Build history of the part. All positions in model axes, mm. A direction names the side the tool comes from. Round coordinates to 2 decimals unless told otherwise and drop trailing zeros. Order: outer loops, then holes, each group sorted by start corner. A loop starts at its lowest first (then second) coordinate and runs counter-clockwise, first axis right, second up. Notation, with made-up numbers: (68.5, 11.5) -> (88.5, 11.5) arc R20 ccw to (88.5, 41.5) -> close; hole circle Ø10 at (76, -27). An arc over 180 degrees is marked (long way). Use a Markdown table: item, result. Add a question column.
Item 1: Two-plate mould, pull along X, no slides. Class faces 5 (the face through (-2.3, 2, -15)), 6 (the face through (-20.94, 1.99, -0.69)), 7 (the face through (19.706, 1.993, -7.112)): released by +X, released by -X, zero draft, split by the parting line, or undercut.
Item 2: Probe L1, parallel to Z at x = -0.5, y = -0.3; L2, parallel to Z at x = -2.5, y = 1; L3, parallel to Z at x = 5, y = 1.9. List the from-to ranges inside material, lowest first.
Item 3: Slice it at C-C, the plane x = 0. State how many separate pieces and enclosed holes the cut face has, plus the area to 3 significant figures.
Item 4: Slice it at D-D, the plane y = -0.6. Give the cut face in (x, z), plus the area to 3 significant figures.
Item 5: 3-axis set-ups, long thin cutter, end or side, ignore diameter. For faces 1 (the face through (-8.53, -0.28, -8.44)), 2 (the face through (19.68, 1.99, 7.18)), 3 (the face through (15, 2, 4.796)), 4 (the face through (3.3, 2, 16)): which of +Z, -Z, +X, -X, +Y, -Y reach the whole face in a straight line?
Item 6: Pin check, flat tips, straight feed: pin 1 (2 mm diameter, centred on x = -3.5, y = 0, fed in from +Z); pin 2 (1.2 mm diameter, centred on x = -2, y = 0, fed in from +Z); pin 3 (19.5 mm diameter, centred on x = -3.5, z = 0.5, fed in from +Y); pin 4 (3 mm diameter, centred on x = 8, z = -14.5, fed in from -Y). Stop position of each tip, or through.
Item 7: Slice it at A-A, the plane x = -17. Give the cut face in (y, z).
from build123d import *

# Parameters (mm, degrees)
SKETCH2_W               = 4.6
SKETCH2_H               = 1.8
WATCH_POSITIONER_DEPTH  = 1
WATCH_HOLDER_V2_DEPTH   = 4
CHAMFER1_SIZE           = 0.6
CUT_EXTRUDE1_DEPTH      = 30.733062405
CUT_EXTRUDE1_DEPTH_BACK = 30.733062405
CHAMFER2_SIZE           = 1


with BuildPart() as part:
    # Front → Base (revolve)
    with BuildSketch(Plane.XY, mode=Mode.PRIVATE) as base_sk:
        Polygon((0, 2.5), (-20.95, 2.5), (-20.95, 1.5), (-13.5, 1.5), (-13.5, -2.5), (0, -2.5), align=None)
    revolve(base_sk.sketch.rotate(Axis((0, 0, 0), (0, 1, 0)), 270), axis=Axis((0, 0, 0), (0, 1, 0)))

    # Sketch2 → Watch Positioner (cut)
    with BuildSketch(Plane(origin=(0, 2.5, 0), x_dir=(1, 0, 0), z_dir=(0, 1, 0))):
        with BuildLine():
            Line((12.3, -4.208325083), (12.3, 4.208325083))
            ThreePointArc((12.3, 4.208325083), (9.192388155, 9.192388155), (4.208325083, 12.3))
            Line((4.208325083, 12.3), (-4.208325083, 12.3))
            ThreePointArc((-4.208325083, 12.3), (-9.192388155, 9.192388155), (-12.3, 4.208325083))
            Line((-12.3, 4.208325083), (-12.3, -4.208325083))
            ThreePointArc((-12.3, -4.208325083), (-9.192388155, -9.192388155), (-4.208325083, -12.3))
            Line((-4.208325083, -12.3), (4.208325083, -12.3))
            ThreePointArc((4.208325083, -12.3), (9.192388155, -9.192388155), (12.3, -4.208325083))
        make_face()
        with Locations((0, 15)):
            Rectangle(SKETCH2_W, SKETCH2_H)
        with Locations((0, -15)):
            Rectangle(SKETCH2_W, SKETCH2_H)
    extrude(amount=-WATCH_POSITIONER_DEPTH, mode=Mode.SUBTRACT)

    # Sketch4 → Watch Holder v2 (cut)
    with BuildSketch(Plane(origin=(0, 2.5, 0), x_dir=(1, 0, 0), z_dir=(0, 1, 0))):
        with BuildLine():
            Line((4.795831523, -11), (-4.795831523, -11))
            ThreePointArc((-4.795831523, -11), (-8.485281374, -8.485281374), (-11, -4.795831523))
            Line((-11, -4.795831523), (-11, 4.795831523))
            ThreePointArc((-11, 4.795831523), (-8.485281374, 8.485281374), (-4.795831523, 11))
            Line((-4.795831523, 11), (4.795831523, 11))
            ThreePointArc((4.795831523, 11), (8.485281374, 8.485281374), (11, 4.795831523))
            Line((11, 4.795831523), (21.95, 4.795831523))
            Line((21.95, 4.795831523), (21.95, -4.795831523))
            Line((21.95, -4.795831523), (11, -4.795831523))
            ThreePointArc((11, -4.795831523), (8.485281374, -8.485281374), (4.795831523, -11))
        make_face()
        with BuildLine():
            Line((15.294471223, 9.395831523), (19.837359955, 9.395831523))
            ThreePointArc((19.837359955, 9.395831523), (17.942483085, 12.643963015), (15.520993847, 15.520993847))
            Line((15.520993847, 15.520993847), (12.692566722, 12.692566722))
            ThreePointArc((12.692566722, 12.692566722), (14.090269301, 11.120558036), (15.294471223, 9.395831523))
        make_face()
        with BuildLine():
            Line((15.520993847, -15.520993847), (12.692566722, -12.692566722))
            ThreePointArc((12.692566722, -12.692566722), (14.090269301, -11.120558036), (15.294471223, -9.395831523))
            Line((15.294471223, -9.395831523), (19.837359955, -9.395831523))
            ThreePointArc((19.837359955, -9.395831523), (17.942483085, -12.643963015), (15.520993847, -15.520993847))
        make_face()
    extrude(amount=-WATCH_HOLDER_V2_DEPTH, mode=Mode.SUBTRACT)

    # Chamfer1
    chamfer1_edges = [part.edges().sort_by_distance(p)[0] for p in [
        (0, 1.5, 11),
        (8.485281374, 1.5, 8.485281374),
        (-8.485281374, 1.5, 8.485281374),
        (-11, 1.5, 0),
        (-8.485281374, 1.5, -8.485281374),
        (0, 1.5, -11),
        (8.485281374, 1.5, -8.485281374),
    ]]
    chamfer(chamfer1_edges, length=CHAMFER1_SIZE)

    # Sketch5 → Cut-Extrude1 (cut, two sides: drawn at the far end of the back side and taken through both)
    with BuildSketch(Plane(origin=(0, 0, 0), x_dir=(1, 0, 0), z_dir=(0, 1, 0)).offset(-CUT_EXTRUDE1_DEPTH_BACK)):
        with BuildLine():
            Line((-12.296968735, 14.418289078), (-9.492775288, 11.614095631))
            ThreePointArc((-9.492775288, 11.614095631), (-6.572021243, 13.483639597), (-3.3, 14.632498078))
            Line((-3.3, 14.632498078), (-3.3, 16.9))
            Line((-3.3, 16.9), (3.3, 16.9))
            Line((3.3, 16.9), (3.3, 14.632498078))
            ThreePointArc((3.3, 14.632498078), (6.344822846, 13.592027923), (9.097684458, 11.926111583))
            Line((9.097684458, 11.926111583), (11.910622272, 14.739049396))
            ThreePointArc((11.910622272, 14.739049396), (-0.251073083, 18.948336663), (-12.296968735, 14.418289078))
        make_face()
        with BuildLine():
            Line((-14.418289078, 12.296968735), (-11.614095631, 9.492775288))
            ThreePointArc((-11.614095631, 9.492775288), (-13.192625168, 7.138251969), (-14.3, 4.52879675))
            Line((-14.3, 4.52879675), (-14.3, 1.5))
            Line((-14.3, 1.5), (-18.890539961, 1.5))
            ThreePointArc((-18.890539961, 1.5), (-17.507517141, 7.251851043), (-14.418289078, 12.296968735))
        make_face()
        with BuildLine():
            Line((-18.890539961, -1.5), (-14.3, -1.5))
            Line((-14.3, -1.5), (-14.3, -4.52879675))
            ThreePointArc((-14.3, -4.52879675), (-13.192625168, -7.138251969), (-11.614095631, -9.492775288))
            Line((-11.614095631, -9.492775288), (-14.418289078, -12.296968735))
            ThreePointArc((-14.418289078, -12.296968735), (-17.507517141, -7.251851043), (-18.890539961, -1.5))
        make_face()
        with BuildLine():
            Line((9.097684458, -11.926111583), (11.910622272, -14.739049396))
            ThreePointArc((11.910622272, -14.739049396), (-0.251073083, -18.948336663), (-12.296968735, -14.418289078))
            Line((-12.296968735, -14.418289078), (-9.492775288, -11.614095631))
            ThreePointArc((-9.492775288, -11.614095631), (-6.572021243, -13.483639597), (-3.3, -14.632498078))
            Line((-3.3, -14.632498078), (-3.3, -16.9))
            Line((-3.3, -16.9), (3.3, -16.9))
            Line((3.3, -16.9), (3.3, -14.632498078))
            ThreePointArc((3.3, -14.632498078), (6.344822846, -13.592027923), (9.097684458, -11.926111583))
        make_face()
    extrude(amount=CUT_EXTRUDE1_DEPTH + CUT_EXTRUDE1_DEPTH_BACK, mode=Mode.SUBTRACT)

    # Chamfer2
    chamfer2_edges = [part.edges().sort_by_distance(p)[0] for p in [
        (8.968295761, 2.5, 9.411146112),
    ]]
    chamfer(chamfer2_edges, length=CHAMFER2_SIZE - 0.0001)  # a hair under: the kernel refuses the full size
    chamfer2_2_edges = [part.edges().sort_by_distance(p)[0] for p in [
        (8.968295761, 2.5, -9.411146112),
    ]]
    chamfer(chamfer2_2_edges, length=CHAMFER2_SIZE - 0.0001)  # a hair under: the kernel refuses the full size
    chamfer2_3_edges = [part.edges().sort_by_distance(p)[0] for p in [
        (-9.192388155, 2.5, 9.192388155),
    ]]
    chamfer(chamfer2_3_edges, length=CHAMFER2_SIZE - 0.0001)  # a hair under: the kernel refuses the full size
    chamfer2_4_edges = [part.edges().sort_by_distance(p)[0] for p in [
        (-9.192388155, 2.5, -9.192388155),
    ]]
    chamfer(chamfer2_4_edges, length=CHAMFER2_SIZE - 0.0001)  # a hair under: the kernel refuses the full size
    chamfer2_5_edges = [part.edges().sort_by_distance(p)[0] for p in [
        (0, 2.5, 12.3),
    ]]
    chamfer(chamfer2_5_edges, length=CHAMFER2_SIZE - 0.0001)  # a hair under: the kernel refuses the full size
    chamfer2_6_edges = [part.edges().sort_by_distance(p)[0] for p in [
        (0, 2.5, -12.3),
    ]]
    chamfer(chamfer2_6_edges, length=CHAMFER2_SIZE - 0.0001)  # a hair under: the kernel refuses the full size
    chamfer2_7_edges = [part.edges().sort_by_distance(p)[0] for p in [
        (-12.3, 2.5, 0),
    ]]
    chamfer(chamfer2_7_edges, length=CHAMFER2_SIZE - 0.0001)  # a hair under: the kernel refuses the full size


solid = part.part
Check sheet entries:
| question | item | result |
|---|---|---|
| 1 | face 5 | undercut |
| 1 | face 6 | split by the parting line |
| 1 | face 7 | released by +X |
| 2 | L1 | -13.49 to -11, 11 to 13.49 |
| 2 | L2 | -13.27 to -11.1, 11.1 to 13.27 |
| 2 | L3 | -20.34 to -18.28, -14.14 to -12.43, 12.43 to 14.14, 18.28 to 20.34 |
| 3 | separate pieces | 5 |
| 3 | enclosed holes | 0 |
| 3 | area | 50.2 mm2 |
| 4 | outline | (-11, -4.8) -> (-11, 4.8) arc R12 cw to (-4.8, 11) -> (4.8, 11) arc R12 cw to (11, 4.8) -> (12.62, 4.8) arc R13.5 ccw (long way) to (12.62, -4.8) -> (11, -4.8) arc R12 cw to (4.8, -11) -> (-4.8, -11) arc R12 cw to start |
| 4 | area | 125 mm2 |
| 5 | face 1 | +Y |
| 5 | face 2 | +Z, +X, +Y, -Y |
| 5 | face 3 | +X, +Y |
| 5 | face 4 | +Y, -Y |
| 6 | pin 1 | z = 13.27 |
| 6 | pin 2 | z = 13.43 |
| 6 | pin 3 | y = 2.45 |
| 6 | pin 4 | through |
| 7 | outline | (1.5, -12.24) -> (2.5, -12.24) -> (2.5, -8.37) -> (1.5, -8.37) -> close; (1.5, -1.5) -> (2.5, -1.5) -> (2.5, 1.5) -> (1.5, 1.5) -> close; (1.5, 8.37) -> (2.5, 8.37) -> (2.5, 12.24) -> (1.5, 12.24) -> close |
